Autodesk Inventor part; units mm, degrees
ref_plane "YZ Plane" through (0, 0, 0) normal (1, 0, 0) x (0, 1, 0)
ref_plane "XZ Plane" through (0, 0, 0) normal (0, 1, 0) x (-1, 0, 0)
ref_plane "XY Plane" through (0, 0, 0) normal (0, 0, 1) x (1, 0, 0)
sketch "スケッチ1" plane through (0, 0, 0) normal (0, 1, 0) x (-1, 0, 0)
  line L0 (-130, -30) -> (130, -30)
  line L1 (130, -30) -> (130, 30)
  line L2 (130, 30) -> (-130, 30)
  line L3 (-130, 30) -> (-130, -30)
  line L4 (-130, -30) -> (130, 30) construction
  line L5 (130, -30) -> (-130, 30) construction
  circle A0 centre (-28, -20) radius 2.6
  circle A1 centre (-20, -20) radius 2.6
  circle A2 centre (20, -20) radius 2.6
  circle A3 centre (28, -20) radius 2.6
  circle A4 centre (-28, 20) radius 2.6
  circle A5 centre (-20, 20) radius 2.6
  circle A6 centre (20, 20) radius 2.6
  circle A7 centre (28, 20) radius 2.6
  point P0 (0, 0)
  dimension "d0" = 260
  dimension "d1" = 60
  dimension "d2" = 5.2
  dimension "d4" = 5.2
  dimension "d5" = 8
  dimension "d6" = 5.2
  dimension "d7" = 40
  dimension "d8" = 5.2
  dimension "d9" = 8
  dimension "d10" = 5.2
  dimension "d12" = 5.2
  dimension "d13" = 5.2
  dimension "d14" = 5.2
  dimension "d16" = 40
  dimension "d17" = 8
  dimension "d18" = 8
  dimension "d20" = 10
  dimension "d21" = 158
  dimension "d22" = 50
  dimension "d23" = 158
extrude "押し出し1" add sketch "スケッチ1" along normal blind 2
sketch "スケッチ2" plane through (0, 0, 0) normal (0, -1, 0) x (1, 0, 0)
  circle A0 centre (-100, 0) radius 12
  circle A1 centre (100, 0) radius 12
  line L0 (-130, -30) -> (-130, 30)
  line L1 (130, 30) -> (130, -30)
  point P0 (0, 0)
  dimension "d26" = 24
  dimension "d27" = 24
  dimension "d28" = 30
  dimension "d29" = 30
extrude "押し出し2" cut sketch "スケッチ2" against normal blind 10
sketch "スケッチ3" plane through (0, 0, 0) normal (0, -1, 0) x (1, 0, 0)
  circle A0 centre (-100, 0) radius 12
  circle A1 centre (-100, 17) radius 2.1
  circle A2 centre (-83, 0) radius 2.1
  circle A3 centre (-100, -17) radius 2.1
  circle A4 centre (-117, 0) radius 2.1
  circle A5 centre (100, 0) radius 12
  circle A6 centre (100, 17) radius 2.1
  circle A7 centre (117, 0) radius 2.1
  circle A8 centre (83, 0) radius 2.1
  circle A9 centre (100, -17) radius 2.1
  point P0 (0, 0)
  dimension "d33" = 4.2
  dimension "d34" = 4.2
  dimension "d35" = 4.2
  dimension "d36" = 4.2
  dimension "d38" = 4.2
  dimension "d39" = 4.2
  dimension "d40" = 4.2
  dimension "d41" = 4.2
extrude "押し出し3" cut sketch "スケッチ3" against normal blind 10 contours A1 | A2 | A3 | A4 | A6 | A7 | A8 | A9
properties part number "UpperArm2"
Can you work these out from the model? Positions are in its coordinate system, mm. Round coordinates to 2 decimals unless told otherwise and drop trailing zeros. Loops run counter-clockwise (first coordinate to the right, second up) from the corner with the lowest first, then second, coordinate; pieces in that order, holes last. Notation, with made-up numbers: (65.5, -5) - (113.5, -5) arc R17 cw to (113.5, 7) - close; hole circle Ø10 at (0.25, 84.5). An arc over 180 degrees is marked (long way). Write item = value, one per line. Start each with the question number.
(1) If we section it at A-A (y = 1.45): Give the number of separate pieces and of enclosed holes in the cut face, and give its area (3 significant figures).
(2) If we section it at B-B (x = 28): Please give me the cut outline in (y, z).
(3) If we mould it in two halves opening along X, with no side actions, what happens to faces 1 (the face through (2, 2, 0)), 2 (the face through (97.9, 0.99, 17.09))? For each: released by +X, released by -X, zero draft, split by the parting line, or undercut.
(4) If we section it at C-C (z = 9): Please give me the cut outline in (x, y).
(5) If I drill on probe 1 along Z at (x, y) = (-20, 1.5); probe 2 along X at (y, z) = (1.25, -20.5); probe 3 along Z at (x, y) = (100, 1.55), over which ranges is the centre line in solid material (lowest first)? Write a range as [from, to].
Ans:
q1.separate_pieces = 1
q1.enclosed_holes = 18
q1.area = 14,400 mm²
q2.outline = (0, -30) - (2, -30) - (2, -22.6) - (0, -22.6) - close; (0, -17.4) - (2, -17.4) - (2, 17.4) - (0, 17.4) - close; (0, 22.6) - (2, 22.6) - (2, 30) - (0, 30) - close
q3.face_1 = zero draft
q3.face_2 = undercut
q4.outline = (-130, 0) - (-107.94, 0) - (-107.94, 2) - (-130, 2) - close; (-92.06, 0) - (92.06, 0) - (92.06, 2) - (-92.06, 2) - close; (107.94, 0) - (130, 0) - (130, 2) - (107.94, 2) - close
q5.probe_1 = [-30, -22.6], [-17.4, 17.4], [22.6, 30]
q5.probe_2 = [-130, -30.55], [-25.45, -22.55], [-17.45, 17.45], [22.55, 25.45], [30.55, 130]
q5.probe_3 = [-30, -19.1], [-14.9, -12], [12, 14.9], [19.1, 30]
